```python
from build123d import *

# Parameters (mm, degrees)
SKETCH_1_W      = 42
SKETCH_1_H      = 42
EXTRUDE_1_DEPTH = 51
SKETCH_2_R      = 11
EXTRUDE_2_DEPTH = 2
EXTRUDE_3_DEPTH = 20.5
CHAMFER_1_SIZE  = 3


with BuildPart() as part:
    # 草图1 → 凸台-拉伸1 (new body)
    with BuildSketch(Plane.XY):
        Rectangle(SKETCH_1_W, SKETCH_1_H)
    extrude(amount=EXTRUDE_1_DEPTH)

    # 草图2 → 凸台-拉伸2 (add)
    with BuildSketch(Plane.XY.offset(51)):
        Circle(SKETCH_2_R)
    extrude(amount=EXTRUDE_2_DEPTH)

    # 草图3 → 凸台-拉伸3 (add)
    with BuildSketch(Plane.XY.offset(53)):
        with BuildLine():
            Line((-1.601826622, 2.315848528), (1.601826622, 2.315848528))
            ThreePointArc((1.601826622, 2.315848528), (0, -2.815848528), (-1.601826622, 2.315848528))
        make_face()
    extrude(amount=EXTRUDE_3_DEPTH)

    # 倒角1
    chamfer_1_edges = [part.edges().sort_by_distance(p)[0] for p in [
        (21, -21, 25.5),
        (-21, -21, 25.5),
        (-21, 21, 25.5),
        (21, 21, 25.5),
    ]]
    chamfer(chamfer_1_edges, length=CHAMFER_1_SIZE)


solid = part.part
```
Source: CAD feature listing. Evaluate the final solid. Frame: model axes, mm. A direction names the side the tool comes from. Round coordinates to 2 decimals unless told otherwise and drop trailing zeros. Order: outer loops, then holes, each group sorted by start corner. A loop starts at its lowest first (then second) coordinate and runs counter-clockwise, first axis right, second up. Notation, with made-up numbers: (58, 64) -> (91, 64) arc R25 cw to (91, 89) -> close; hole circle Ø5 at (-35.75, 2.25). An arc over 180 degrees is marked (long way). Use CSV: the item, a comma, the result in double quotes.
(1) Access query for faces 1 (the face through (0, 21, 25)), 2 (the face through (0, 2.316, 63)), 3 (the face through (-2.38, -10.74, 51.99)). Directions: +Z, -Z, +X, -X, +Y, -Y. A direction counts if a zero-diameter tool reaches every point of the face in a straight line with its end or side. Return the directions, or none.
Report:
face 1,"+Z, -Z, +X, -X, +Y"
face 2,"+Z, +X, -X, +Y"
face 3,"+Z"
(2) Ray query, L1, parallel to Z at x = -17.5, y = -4.5; L2, parallel to Z at x = 9, y = 3; L3, parallel to Y at x = 19, z = 19. Return the intervals inside material, ascending.
Report:
L1,"0 to 51"
L2,"0 to 53"
L3,"-20 to 20"
(3) Section B-B on y = 0. Return the cut outline in (x, z).
Report:
outline,"(-21, 0) -> (21, 0) -> (21, 51) -> (11, 51) -> (11, 53) -> (2.82, 53) -> (2.82, 73.5) -> (-2.82, 73.5) -> (-2.82, 53) -> (-11, 53) -> (-11, 51) -> (-21, 51) -> close"
(4) Section A-A on x = 0. Return the cut outline in (y, z), and give its area (3 significant figures).
Report:
outline,"(-21, 0) -> (21, 0) -> (21, 51) -> (11, 51) -> (11, 53) -> (2.32, 53) -> (2.32, 73.5) -> (-2.82, 73.5) -> (-2.82, 53) -> (-11, 53) -> (-11, 51) -> (-21, 51) -> close"
area,"2,290 mm^2"
(5) Section D-D on x = -4.5. Return the cut outline in (y, z).
Report:
outline,"(-21, 0) -> (21, 0) -> (21, 51) -> (10.04, 51) -> (10.04, 53) -> (-10.04, 53) -> (-10.04, 51) -> (-21, 51) -> close"
(6) First-contact query: pin 1 Ø3 at (x, y) = (4.5, 5.5) entering from +Z; pin 2 Ø3 at (x, y) = (16.5, -16.5) entering from -Z; pin 3 Ø1.5 at (x, y) = (-8, -11) entering from +Z; pin 4 Ø2.5 at (x, z) = (-0.5, 60) entering from +Y. Flat tips, straight axial feed; report the tip coordinate or a pass-through.
Report:
pin 1,"z = 53"
pin 2,"z = 0"
pin 3,"z = 51"
pin 4,"y = 2.32"
(7) Section C-C on z = 64.5. Return the cut outline in (x, y).
Report:
outline,"(-1.6, 2.32) arc R2.82 ccw (long way) to (1.6, 2.32) -> close"
